Verification items for the finished model (mm, model axes). Face numbers are marked on the shaded views. A direction names the side the tool comes from. Give positions to 0.01 mm unless a question says otherwise; leave off trailing zeros. Write each loop counter-clockwise with the first axis right and the second up, starting at its lowest first coordinate (ties: lowest second). Pieces come first, ordered by that corner, then holes. Notation, with made-up numbers: (-39.5, 44) - (18.5, 44) arc R14 ccw to (18.5, 50) - close; hole circle Ø8 at (73.5, 59). An arc over 180 degrees is marked (long way). Answer as a JSON object with one key per item and string values. Group by question number.
Item 1: Tool access check on the marked faces 4, 5 and 6. Record the directions out of +Z, -Z, +X, -X, +Y, -Y that give a thin tool (end or side, any length) a straight path to the whole face; none if there is none.
Item 2: Sectioned sample at C-C, the plane y = -3. Record the boundary of the cut face in (x, z).
Item 3: Sectioned sample at A-A, the plane x = 16.5. Record the boundary of the cut face in (y, z).
Item 4: Sectioned sample at B-B, the plane y = -38.1. Record the boundary of the cut face in (x, z).
Item 5: Draft check along X on the marked faces 1, 2 and 3. Enter one of: +X half, -X half, draft (parallel to the pull), parting line (faces both ways), or undercut.
Item 6: Go/stop test with flat-tipped pins: pin 1 (10 mm diameter, centred on x = 16, y = -13.5, fed in from -Z); pin 2 (10 mm diameter, centred on y = -45, z = -8.5, fed in from +X); pin 3 (14.5 mm diameter, centred on x = 69.596, y = -38.1, fed in from -Z); pin 4 (12.5 mm diameter, centred on x = 133, z = -6, fed in from -Y). Record where each tip stops, or that it passes through.
Item 7: Sectioned sample at D-D, the plane x = 113.5. Record the boundary of the cut face in (y, z), and give its area (3 significant figures).
Item 8: Scan lines: line 1 along X through (y, z) = (-36.5, 3); line 2 along Y through (x, z) = (116, -11.5); line 3 along X through (y, z) = (-38.1, 4.25). Record each from-to range of solid material in increasing order. Write a range as [from, to].
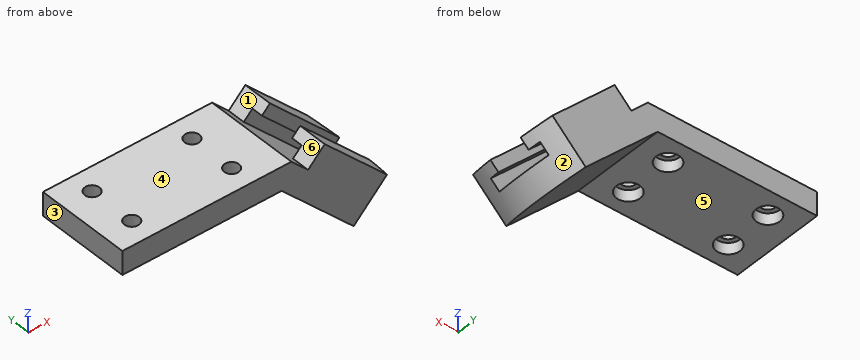
```python
from build123d import *

# Parameters (mm, degrees)
F1_DEPTH       = 50.8
F3_D           = 7.9248
F3_CBORE_D     = 12.7
F3_CBORE_DEPTH = 6.096
F5_DEPTH       = 118.4823439803
F7_DEPTH       = 66.5486543438


with BuildPart() as f1:
    # F0 (on Front) → F1 (new body)
    with BuildSketch(Plane.XZ):
        Polygon((0, 12.7), (0, 0), (85.852, 0), (131.6378767242, -45.7858767242), (149.7304108726, -27.9583640517), (109.0720468209, 12.7), (100.0917906999, 3.7197438789), (91.1115345788, 12.7), align=None)
    extrude(amount=F1_DEPTH)

    # F3 (through all)
    with Locations(Plane(origin=(0, 0, 0), x_dir=(1, 0, 0), z_dir=(0, 0, -1))):
        with Locations((15.748, 12.7), (15.748, 38.1), (69.596, 38.1), (69.596, 12.7)):
            CounterBoreHole(F3_D / 2, F3_CBORE_D / 2, F3_CBORE_DEPTH)

    # F4 (on face) → F5 (cut, through all)
    with BuildSketch(Plane(origin=(60.8860234105, 0, 60.8860234105), x_dir=(0.7071067812, 0, -0.7071067812), z_dir=(0.7071067812, 0, 0.7071067812))):
        with BuildLine():
            ThreePointArc((115.6263461786, 0), (121.9933278239, -25.4), (115.6263461786, -50.8))
            Line((115.6263461786, -50.8), (125.6449376897, -50.8))
            Line((125.6449376897, -50.8), (125.6449376897, 0))
            Line((125.6449376897, 0), (115.6263461786, 0))
        make_face()
    extrude(amount=-F5_DEPTH, mode=Mode.SUBTRACT)

    # F6 (on face) → F7 (cut, through all)
    with BuildSketch(Plane(origin=(48.1860234105, 0, -48.1860234105), x_dir=(0, -1, 0), z_dir=(-0.7071067812, 0, 0.7071067812))):
        Polygon((9.652, 73.405840066), (41.148, 73.405840066), (41.148, 80.009840066), (35.052, 80.009840066), (35.052, 86.105840066), (15.748, 86.105840066), (15.748, 80.009840066), (9.652, 80.009840066), align=None)
    extrude(amount=-F7_DEPTH, mode=Mode.SUBTRACT)


solid = f1.part
```
Geometry check:
{
 "1": {"face 4": "+Z, +X, -X, +Y, -Y", "face 5": "-Z, -X, +Y, -Y", "face 6": "+Z, +Y, -Y"},
 "2": {"outline": "(0, 0) - (85.85, 0) - (125.74, -39.89) - (143.7, -21.93) - (109.07, 12.7) - (100.09, 3.72) - (91.11, 12.7) - (0, 12.7) - close"},
 "3": {"outline": "(-50.8, 0) - (-44.41, 0) - (-44.41, 6.1) - (-41.99, 6.1) - (-41.99, 12.7) - (-50.8, 12.7) - close; (-34.21, 6.1) - (-31.79, 6.1) - (-31.79, 0) - (-19.01, 0) - (-19.01, 6.1) - (-16.59, 6.1) - (-16.59, 12.7) - (-34.21, 12.7) - close; (-8.81, 6.1) - (-6.39, 6.1) - (-6.39, 0) - (0, 0) - (0, 12.7) - (-8.81, 12.7) - close"},
 "4": {"outline": "(0, 0) - (9.4, 0) - (9.4, 6.1) - (11.79, 6.1) - (11.79, 12.7) - (0, 12.7) - close; (19.71, 6.1) - (22.1, 6.1) - (22.1, 0) - (63.25, 0) - (63.25, 6.1) - (65.63, 6.1) - (65.63, 12.7) - (19.71, 12.7) - close; (73.56, 6.1) - (75.95, 6.1) - (75.95, 0) - (85.85, 0) - (128.11, -42.26) - (137.09, -33.28) - (91.11, 12.7) - (73.56, 12.7) - close; (104.76, 8.39) - (141.76, -28.61) - (146.07, -24.3) - (109.07, 12.7) - close"},
 "5": {"face 1": "undercut", "face 2": "+X half", "face 3": "-X half"},
 "6": {"pin 1": "z = 6.1", "pin 2": "x = 135.27", "pin 3": "z = 0", "pin 4": "y = -50.8"},
 "7": {"outline": "(-50.8, -27.65) - (0, -27.65) - (0, 8.27) - (-15.75, 8.27) - (-15.75, -0.35) - (-9.65, -0.35) - (-9.65, -9.69) - (-41.15, -9.69) - (-41.15, -0.35) - (-35.05, -0.35) - (-35.05, 8.27) - (-50.8, 8.27) - close", "area": "1,360 mm^2"},
 "8": {"line 1": "[0, 9.6], [21.89, 63.45], [75.74, 100.81], [110.15, 118.77]", "line 2": "[-50.8, -41.15], [-9.65, 0]", "line 3": "[0, 9.4], [22.1, 63.25], [75.95, 99.56], [108.9, 117.52]"}
}
